Check sheet for the modelled part. Datum: model origin and axes. Units: mm. A direction names the side the tool comes from. Give positions to 0.01 mm unless a question says otherwise; leave off trailing zeros. Write each loop counter-clockwise with the first axis right and the second up, starting at its lowest first coordinate (ties: lowest second). Pieces come first, ordered by that corner, then holes. Notation, with made-up numbers: (2.25, 55) -> (58.25, 55) arc R21 cw to (58.25, 65) -> close; hole circle Ø3 at (60.25, 3.25). An arc over 180 degrees is marked (long way). Use a Markdown table: item, result. Add a question column.
1. Scan lines: probe 1 along Z at (x, y) = (-10.25, 5); probe 2 along Y at (x, z) = (-7.5, -37.5); probe 3 along X at (y, z) = (29, -5.5). Record each from-to range of solid material in increasing order. Write a range as [from, to].
2. Gauge pin test, flat ends, axial feed: P1, Ø7, axis at y = 53.08, z = 1.25, coming from the +X side; P2, Ø3, axis at x = -1, y = 9, coming from the -Z side; P3, Ø12, axis at x = 4, z = 12.5, coming from the +Y side; P4, Ø4, axis at x = -3.589, z = 37.211, coming from the +Y side. Record the tip position at first contact, or that the pin passes through.
3. Release check for a two-part mould opening along Y. For faces 4 (the cylindrical face through (4.131, -0.373, -46.826)), 5 (the cylindrical face through (-11.37, 49.3, 0.06)), 6 (the cylindrical face through (-3.24, 53.574, -17.06)) record: released by +Y, released by -Y, zero draft, split by the parting line, or undercut.
4. Cross-section at D-D (z = 16.5). Enter the section's corners in (x, y), then the cut area to 3 significant figures.
5. Cross-section at A-A (y = 52). Enter the section's corners in (x, z).
6. Cross-section at B-B (z = 0). Enter the section's corners in (x, y), then the cut area to 3 significant figures.
7. Set-up check for faces 1 (the flat face through (-6, 27, -17.423)), 2 (the flat face through (-6, 28, 35.8)), 3 (the flat face through (-6, 28, 36.537)): record each of +Z, -Z, +X, -X, +Y, -Y from which the full face is reachable in a straight line by a thin tool's end or side.
8. Cross-section at C-C (x = 0.75). Enter the section's corners in (y, z), then the cut area to 3 significant figures.
from build123d import *

# Parameters (mm, degrees)
SKETCH1_W                 = 20
SKETCH1_H                 = 101.6
BASE_FLANGE1_DEPTH        = 0.7366
EDGE_FLANGE1_DEPTH        = 50.486713846
EDGE_FLANGE1_START        = 0.7366
EDGE_FLANGE1_FLAT_DEPTH   = 0.7366
CUT_EXTRUDE1_DEPTH        = 245.392554313
CUT_EXTRUDE1_DEPTH_BACK   = 245.392554313
SKETCH9_R                 = 2
CUT_EXTRUDE3_DEPTH        = 248.026355859
CUT_EXTRUDE3_DEPTH_BACK   = 248.026355859
SKETCH11_R                = 3.96875
CUT_EXTRUDE5_DEPTH        = 199.550344579
CUT_EXTRUDE5_DEPTH_BACK   = 199.550344579
SKETCH13_R                = 1.984375
SKETCH13_R_2              = 1.190625
EDGE_FLANGE2_DEPTH        = 54.2634
EDGE_FLANGE2_START        = 0.7366
EDGE_FLANGE2_FLAT_DEPTH   = 0.7366
EDGE_FLANGE2_BEND_DEPTH   = 54.2634
EDGE_FLANGE2_FLAT_2_DEPTH = 0.7366
CUT_EXTRUDE35_DEPTH       = 251.457429571
CUT_EXTRUDE35_DEPTH_BACK  = 251.457429571
SKETCH50_R                = 3.325000001


# Sheet-metal steps are written as plain solids
with BuildPart() as part:
    # Sketch1 → Base-Flange1 (new body)
    with BuildSketch(Plane(origin=(0, 0, 0), x_dir=(1, 0, 0), z_dir=(0, 1, 0))):
        Rectangle(SKETCH1_W, SKETCH1_H)
    extrude(amount=-BASE_FLANGE1_DEPTH)

    # Edge-Flange1 bend section (across the edge) → Edge-Flange1 (add)
    with BuildSketch(Plane(origin=(-11, 0, -15.686713846), x_dir=(1, 0, 0), z_dir=(0, 0, 1))):
        with BuildLine():
            Line((-0.7366, 0.7366), (0, 0.7366))
            ThreePointArc((0, 0.7366), (0.215745145, 0.215745145), (0.7366, 0))
            Line((0.7366, 0), (1, 0))
            Line((1, 0), (1, -0.7366))
            Line((1, -0.7366), (0.7366, -0.7366))
            ThreePointArc((0.7366, -0.7366), (-0.30510971, -0.30510971), (-0.7366, 0.7366))
        make_face()
    extrude(amount=EDGE_FLANGE1_DEPTH)

    # Edge-Flange1 profile (on flange) → Edge-Flange1 flat (add)
    with BuildSketch(Plane.ZY.offset(11).offset(EDGE_FLANGE1_START)):
        with BuildLine():
            ThreePointArc((34.8, 55), (9.556643077, 80.243356923), (-15.686713846, 55))
            Line((-15.686713846, 55), (-15.686713846, 0.7366))
            Line((-15.686713846, 0.7366), (34.8, 0.7366))
            Line((34.8, 0.7366), (34.8, 55))
        make_face()
    extrude(amount=-EDGE_FLANGE1_FLAT_DEPTH)

    # Sketch9 → Cut-Extrude1 (cut, two sides: drawn at the far end of the back side and taken through both)
    with BuildSketch(Plane(origin=(-48.111610167, -124.793980752, 68.826299478), x_dir=(0, 0, -1), z_dir=(1, 0, 0)).offset(-CUT_EXTRUDE1_DEPTH_BACK)):
        with Locations(Location((68.826299478, 136.507533033, 0), (0, 0, 270))):
            Circle(SKETCH9_R)
    extrude(amount=CUT_EXTRUDE1_DEPTH + CUT_EXTRUDE1_DEPTH_BACK, mode=Mode.SUBTRACT)

    # Sketch11 → Cut-Extrude3 (cut, two sides: drawn at the far end of the back side and taken through both)
    with BuildSketch(Plane(origin=(-58.346610167, -124.793980752, 68.826299478), x_dir=(0, 0, -1), z_dir=(1, 0, 0)).offset(-CUT_EXTRUDE3_DEPTH_BACK)):
        with Locations(Location((67.576820433, 177.878571709, 0), (0, 0, 270))):
            Circle(SKETCH11_R)
    extrude(amount=CUT_EXTRUDE3_DEPTH + CUT_EXTRUDE3_DEPTH_BACK, mode=Mode.SUBTRACT)

    # Sketch13 → Cut-Extrude5 (cut, two sides: drawn at the far end of the back side and taken through both)
    with BuildSketch(Plane(origin=(124.911822879, 0, 68.826299478), x_dir=(-0.7071067811865436, 0, 0.7071067811865515), z_dir=(0, 1, 0)).offset(-CUT_EXTRUDE5_DEPTH_BACK)):
        with Locations(Location((68.508410595, -102.424928038, 0), (0, 0, 45))):
            Circle(SKETCH13_R)
        with Locations(Location((68.508410595, -113.219195896, 0), (0, 0, 45))):
            Circle(SKETCH13_R_2)
        with Locations(Location((5.089841868, -165.843496765, 0), (0, 0, 45))):
            Circle(SKETCH13_R)
        with Locations(Location((15.884109726, -165.843496765, 0), (0, 0, 45))):
            Circle(SKETCH13_R_2)
    extrude(amount=CUT_EXTRUDE5_DEPTH + CUT_EXTRUDE5_DEPTH_BACK, mode=Mode.SUBTRACT)

    # Edge-Flange2 bend section (across the edge) → Edge-Flange2 (add)
    with BuildSketch(Plane(origin=(-11, 0.7366, -16.686713846), x_dir=(0, 0, 1), z_dir=(0, 1, 0))):
        with BuildLine():
            Line((-0.7366, 0.7366), (0, 0.7366))
            ThreePointArc((0, 0.7366), (0.215745145, 0.215745145), (0.7366, 0))
            Line((0.7366, 0), (1, 0))
            Line((1, 0), (1, -0.7366))
            Line((1, -0.7366), (0.7366, -0.7366))
            ThreePointArc((0.7366, -0.7366), (-0.30510971, -0.30510971), (-0.7366, 0.7366))
        make_face()
    extrude(amount=EDGE_FLANGE2_DEPTH)

    # Edge-Flange2 profile (on flange) → Edge-Flange2 flat (add)
    with BuildSketch(Plane(origin=(-11, 0, -16.686713846), x_dir=(0, 1, 0), z_dir=(0, 0, -1)).offset(EDGE_FLANGE2_START)):
        with BuildLine():
            Line((50, 9.2634), (0.7366, 9.2634))
            Line((0.7366, 9.2634), (0.7366, 0.7366))
            Line((0.7366, 0.7366), (55, 0.7366))
            Line((55, 0.7366), (55, 4.2634))
            ThreePointArc((55, 4.2634), (53.535533906, 7.798933906), (50, 9.2634))
        make_face()
    extrude(amount=-EDGE_FLANGE2_FLAT_DEPTH)

    # Edge-Flange2 bend section 2 (across the edge) → Edge-Flange2 bend (add)
    with BuildSketch(Plane(origin=(-11, 55, 35.8), x_dir=(0, 0, -1), z_dir=(0, -1, 0))):
        with BuildLine():
            Line((-0.7366, 0.7366), (0, 0.7366))
            ThreePointArc((0, 0.7366), (0.215745145, 0.215745145), (0.7366, 0))
            Line((0.7366, 0), (1, 0))
            Line((1, 0), (1, -0.7366))
            Line((1, -0.7366), (0.7366, -0.7366))
            ThreePointArc((0.7366, -0.7366), (-0.30510971, -0.30510971), (-0.7366, 0.7366))
        make_face()
    extrude(amount=EDGE_FLANGE2_BEND_DEPTH)

    # Edge-Flange2 profile 2 (on flange) → Edge-Flange2 flat 2 (add)
    with BuildSketch(Plane(origin=(-11, 0, 35.8), x_dir=(0, -1, 0), z_dir=(0, 0, 1)).offset(EDGE_FLANGE2_START)):
        with BuildLine():
            ThreePointArc((-50, 9.2634), (-53.535533906, 7.798933906), (-55, 4.2634))
            Line((-55, 4.2634), (-55, 0.7366))
            Line((-55, 0.7366), (-0.7366, 0.7366))
            Line((-0.7366, 0.7366), (-0.7366, 9.2634))
            Line((-0.7366, 9.2634), (-50, 9.2634))
        make_face()
    extrude(amount=-EDGE_FLANGE2_FLAT_2_DEPTH)

    # Sketch50 → Cut-Extrude35 (cut, two sides: drawn at the far end of the back side and taken through both)
    with BuildSketch(Plane(origin=(-69.8634, -124.793980752, 68.826299478), x_dir=(0, 0, -1), z_dir=(1, 0, 0)).offset(-CUT_EXTRUDE35_DEPTH_BACK)):
        with Locations(Location((43.461576529, 148.105383059, 0), (0, 0, 270))):
            Circle(SKETCH50_R)
    extrude(amount=CUT_EXTRUDE35_DEPTH + CUT_EXTRUDE35_DEPTH_BACK, mode=Mode.SUBTRACT)


solid = part.part
Worked answers:
| question | item | result |
|---|---|---|
| 1 | probe 1 | z = [-17.42, -16.69], [35.8, 36.54] |
| 1 | probe 2 | y = [-0.74, 0] |
| 1 | probe 3 | x = [-11.74, -11] |
| 2 | P1 | passes through |
| 2 | P2 | stops at z = -17.42 |
| 2 | P3 | stops at y = 0 |
| 2 | P4 | stops at y = 54.84 |
| 3 | face 4 | zero draft |
| 3 | face 5 | undercut |
| 3 | face 6 | released by +Y |
| 4 | outline | (-11.74, 0.74) arc R1.47 ccw to (-10.26, -0.74) -> (10, -0.74) -> (10, 0) -> (-10.26, 0) arc R0.74 cw to (-11, 0.74) -> (-11, 79.27) -> (-11.74, 79.27) -> close |
| 4 | area | 74.1 mm² |
| 5 | outline | (-11.74, -15.95) arc R1.47 ccw to (-10.26, -17.42) -> (-2.15, -17.42) -> (-2.15, -16.69) -> (-10.26, -16.69) arc R0.74 cw to (-11, -15.95) -> (-11, -2.57) -> (-11.74, -2.57) -> close; (-11.74, 5.07) -> (-11, 5.07) -> (-11, 35.06) arc R0.74 cw to (-10.26, 35.8) -> (-2.15, 35.8) -> (-2.15, 36.54) -> (-10.26, 36.54) arc R1.47 ccw to (-11.74, 35.06) -> close |
| 6 | outline | (-11.74, 0.74) arc R1.47 ccw to (-10.26, -0.74) -> (10, -0.74) -> (10, 0) -> (-10.26, 0) arc R0.74 cw to (-11, 0.74) -> (-11, 9.71) -> (-11.74, 9.71) -> close; (-11.74, 13.71) -> (-11, 13.71) -> (-11, 49.32) -> (-11.74, 49.32) -> close; (-11.74, 56.85) -> (-11, 56.85) -> (-11, 78.36) -> (-11.74, 78.36) -> close |
| 6 | area | 64.9 mm² |
| 7 | face 1 | -Z, +X, -X, +Y |
| 7 | face 2 | +X, +Y |
| 7 | face 3 | +Z, +X, -X, +Y |
| 8 | outline | (-0.74, -50.8) -> (0, -50.8) -> (0, 50.8) -> (-0.74, 50.8) -> close |
| 8 | area | 74.8 mm² |
